Check sheet for the modelled part. Datum: model origin and axes. Units: mm. Coordinates: 2 decimals unless noted, no trailing zeros. Loops run counter-clockwise (first coordinate to the right, second up) from the corner with the lowest first, then second, coordinate; pieces in that order, holes last. Notation, with made-up numbers: M -32.5,78 L -8.5,78 A16 cw -8.5,88 Z; hole C 84,63.5 d4. An arc over 180 degrees is marked long. Write each question's results on one line, items separated by ' | '. Start each with the question number.
Autodesk Inventor part; units mm, degrees
ref_plane "YZ Plane" through (0, 0, 0) normal (1, 0, 0) x (0, 1, 0)
ref_plane "XZ Plane" through (0, 0, 0) normal (0, 1, 0) x (-1, 0, 0)
ref_plane "XY Plane" through (0, 0, 0) normal (0, 0, 1) x (1, 0, 0)
sketch "スケッチ1" plane through (0, 0, 0) normal (0, 1, 0) x (-1, 0, 0)
  circle A0 centre (0, 0) radius 13
  dimension "d0" = 26
extrude "押し出し1" add sketch "スケッチ1" along normal blind 35
fillet "フィレット1" radius 1 2 edges at (13, 0, 0) (13, 35, 0)
sketch "スケッチ2" plane through (0, 35, 0) normal (0, 1, 0) x (1, 0, 0)
  circle A0 centre (0, 0) radius 12
extrude "押し出し2" cut sketch "スケッチ2" against normal blind 1
properties part number "Capacitor"
1) Thickness scan on probe 1 along Z at (x, y) = (0, 34.35); probe 2 along Z at (x, y) = (0, 34.7); probe 3 along Y at (x, z) = (-9.5, -6.5). Record the ranges inside material, lowest first.
2) Section check A-A (x = 0). Enter the section's corners in (y, z).
3) Gauge pin test, flat ends, axial feed: P1, Ø6, axis at x = 8, z = 0, coming from the +Y side; P2, Ø10, axis at y = 8.5, z = 9.5, coming from the -X side. Record the tip position at first contact, or that the pin passes through.
4) Release check for a two-part mould opening along Z. For faces 1 (the cylindrical face through (10.316, 17.269, 7.91)), 2 (the flat face through (0, 0, 0)), 3 (the cylindrical face through (-11.99, 34.51, -0.53)) record: +Z half, -Z half, draft (parallel to the pull), parting line (faces both ways), or undercut.
5) Section check B-B (z = 0). Enter the section's corners in (x, y), then the cut area to 3 significant figures.
6) Section check C-C (y = 7.5). Enter the section's corners in (x, z), then the cut area to 3 significant figures.
Return value:
1) probe 1: z = -12.94 to -12, 12 to 12.94 | probe 2: z = -12.71 to -12, 12 to 12.71 | probe 3: y = 0 to 34
2) outline: M 0,-12 A1 ccw 1,-13 L 34,-13 A1 ccw 35,-12 L 34,-12 L 34,12 L 35,12 A1 ccw 34,13 L 1,13 A1 ccw 0,12 Z
3) P1: stops at y = 34 | P2: stops at x = -12.2
4) face 1: parting line | face 2: draft | face 3: undercut
5) outline: M -13,1 A1 ccw -12,0 L 12,0 A1 ccw 13,1 L 13,34 A1 ccw 12,35 L 12,34 L -12,34 L -12,35 A1 ccw -13,34 Z | area: 885 mm2
6) outline: C 0,0 d26 | area: 531 mm2
